```python
from build123d import *

# Parameters (mm, degrees)
BOSS_EXTRUDE1_DEPTH = 12.7
FILLET3_R           = 6.35
FILLET4_R           = 6.35


with BuildPart() as part:
    # Sketch5 → Boss-Extrude1 (new body)
    with BuildSketch(Plane.XY):
        with BuildLine():
            Line((0, 0), (12.7, 0))
            Line((12.7, 0), (12.7, 203.2))
            ThreePointArc((12.7, 203.2), (-34.29, 250.19), (-81.28, 203.2))
            Line((-81.28, 203.2), (-81.28, 152.4))
            Line((-81.28, 152.4), (-68.58, 152.4))
            Line((-68.58, 152.4), (-68.58, 203.2))
            ThreePointArc((-68.58, 203.2), (-34.29, 237.49), (0, 203.2))
            Line((0, 203.2), (0, 0))
        make_face()
    extrude(amount=BOSS_EXTRUDE1_DEPTH)

    # Fillet3
    fillet3_edges = [part.edges().sort_by_distance(p)[0] for p in [
        (-68.58, 152.4, 6.35),
    ]]
    fillet(fillet3_edges, radius=FILLET3_R)

    # Fillet4
    fillet4_edges = [part.edges().sort_by_distance(p)[0] for p in [
        (-81.28, 152.4, 6.35),
    ]]
    fillet(fillet4_edges, radius=FILLET4_R - 0.0001)  # a hair under: the kernel refuses the full size


solid = part.part
```
The listing builds one solid part. Answer for the finished solid, in the listing's coordinates (mm). A direction names the side the tool comes from. Coordinates: 2 decimals unless noted, no trailing zeros. Write each loop counter-clockwise with the first axis right and the second up, starting at its lowest first coordinate (ties: lowest second). Pieces come first, ordered by that corner, then holes. Notation, with made-up numbers: M -20.75,-20.5 L 13.25,-20.5 A21 cw 13.25,15.5 Z; hole C -10,84 d6. An arc over 180 degrees is marked long. Use a Markdown table: item, result. Add a question column.
1. For a pull along X with two mould halves and no side action, classify faces 1 (the cylindrical face through (-70.5, 154.2, 6.4)), 2 (the flat face through (6, 0, 6)), 3 (the flat face through (12.7, 100, 6)), 4 (the flat face through (0, 103, 6)) as +X half, -X half, draft (parallel to the pull), parting line (faces both ways), or undercut.
2. Given P1, Ø1, axis at x = -21, z = 3, coming from the +Y side; P2, Ø6.5, axis at y = 130, z = 3.5, coming from the -X side; P3, Ø1, axis at x = -56.5, z = 5, coming from the +Y side, each flat-ended and moving along its own axis, determine where each tip first touches the part or whether it passes through.
3. Which of the six approach directions +Z, -Z, +X, -X, +Y, -Y give full straight-line access (tool end or side, diameter ignored) to faces 5 (the flat face through (-68.58, 181, 6)), 6 (the flat face through (0.3, 144.2, 0))?
4. Section D-D (y = 53) is taken. Give the vertices of the cut face in (x, z).
5. Section A-A (y = 163) is taken. Give the vertices of the cut face in (x, z).
6. Straight lines are drawn through the part: line 1 along X through (y, z) = (182, 7.5); line 2 along X through (y, z) = (52.5, 2); line 3 along Y through (x, z) = (-32.5, 1). For each, find the intervals that lie inside material, in ascending order. Write a range as [from, to].
7. Section C-C (x = -34.29) is taken. Give the vertices of the cut face in (y, z).
Data:
| question | item | result |
|---|---|---|
| 1 | face 1 | undercut |
| 1 | face 2 | draft |
| 1 | face 3 | +X half |
| 1 | face 4 | undercut |
| 2 | P1 | stops at y = 248.42 |
| 2 | P2 | stops at x = 0 |
| 2 | P3 | stops at y = 244.87 |
| 3 | face 5 | +Z, -Z, -Y |
| 3 | face 6 | -Z, +X, -X, +Y, -Y |
| 4 | outline | M 0,0 L 12.7,0 L 12.7,12.7 L 0,12.7 Z |
| 5 | outline | M -81.28,0 L -68.58,0 L -68.58,12.7 L -81.28,12.7 Z; M 0,0 L 12.7,0 L 12.7,12.7 L 0,12.7 Z |
| 6 | line 1 | x = [-81.28, -68.58], [0, 12.7] |
| 6 | line 2 | x = [0, 12.7] |
| 6 | line 3 | y = [237.44, 250.16] |
| 7 | outline | M 237.49,0 L 250.19,0 L 250.19,12.7 L 237.49,12.7 Z |
